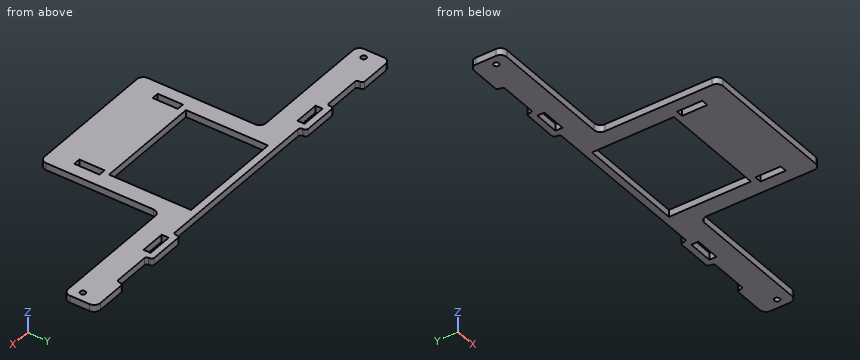
```python
from build123d import *

# Parameters (mm, degrees)
SKETCH_1_W               = 325
SKETCH_1_H               = 110
SKETCH_1_R               = 2.1
EXTRUDE_1_DEPTH          = 5.6
EXTRUDE_2_DEPTH          = 5.6
SKETCH_2_W               = 85
SKETCH_2_H               = 65
SKETCH_2_W_2             = 5.6
SKETCH_2_H_2             = 20
SKETCH_2_W_3             = 20
SKETCH_2_H_3             = 5.6
CUT_EXTRUDE_1_DEPTH      = 176.331029769
SKETCH_4_W               = 106.4
SKETCH_4_H               = 95
SKETCH_4_R               = 2.1
CUT_EXTRUDE_2_DEPTH      = 176.331029769
CUT_EXTRUDE_3_DEPTH      = 176.331029769
CUT_EXTRUDE_3_DEPTH_BACK = 176.331029769
SKETCH_5_W               = 140
SKETCH_5_H               = 5
SKETCH_5_W_2             = 32.5
FILLET_1_R               = 5
FILLET_2_R               = 2


with BuildPart() as part:
    # ｽｹｯﾁ1 → ﾎﾞｽ - 押し出し1 (new body)
    with BuildSketch(Plane.XY):
        Rectangle(SKETCH_1_W, SKETCH_1_H)
        with Locations((155, 50)):
            Circle(SKETCH_1_R, mode=Mode.SUBTRACT)
        with Locations(Location((155, -50, 0), (0, 0, 180))):
            Circle(SKETCH_1_R, mode=Mode.SUBTRACT)
        with Locations(Location((-155, 50, 0), (0, 0, 180))):
            Circle(SKETCH_1_R, mode=Mode.SUBTRACT)
        with Locations((-155, -50)):
            Circle(SKETCH_1_R, mode=Mode.SUBTRACT)
    extrude(amount=EXTRUDE_1_DEPTH)

    # ｽｹｯﾁ3 → ﾎﾞｽ - 押し出し2 (add)
    with BuildSketch(Plane.XY.offset(5.6)):
        Polygon((-162.5, 65.6), (-162.5, 55), (-95, 55), (-95, 60.6), (-75, 60.6), (-75, 55), (0, 55), (0, 65.6), align=None)
        Polygon((162.5, 65.6), (0, 65.6), (0, 55), (75, 55), (75, 60.6), (95, 60.6), (95, 55), (162.5, 55), align=None)
    extrude(amount=-EXTRUDE_2_DEPTH)

    # ｽｹｯﾁ2 → ｶｯﾄ - 押し出し1 (cut, through all)
    with BuildSketch(Plane.XY.offset(5.6)):
        with Locations((0, 22.5)):
            Rectangle(SKETCH_2_W, SKETCH_2_H)
        with Locations((-43.3, -25)):
            Rectangle(SKETCH_2_W_2, SKETCH_2_H_2)
        with Locations((43.3, -25)):
            Rectangle(SKETCH_2_W_2, SKETCH_2_H_2)
        with Locations((85, 57.8)):
            Rectangle(SKETCH_2_W_3, SKETCH_2_H_3)
        with Locations((-85, 57.8)):
            Rectangle(SKETCH_2_W_3, SKETCH_2_H_3)
    extrude(amount=-CUT_EXTRUDE_1_DEPTH, mode=Mode.SUBTRACT)

    # ｽｹｯﾁ4 → ｶｯﾄ - 押し出し2 (cut, through all)
    # profile 1 of 2: a face of its own
    with BuildSketch(Plane.XY.offset(5.6)):
        with Locations((-109.3, -7.5)):
            Rectangle(SKETCH_4_W, SKETCH_4_H)
        with Locations((-155, -50)):
            Circle(SKETCH_4_R, mode=Mode.SUBTRACT)
    # profile 2 of 2: a face of its own
    with BuildSketch(Plane.XY.offset(5.6)):
        with Locations((109.3, -7.5)):
            Rectangle(SKETCH_4_W, SKETCH_4_H)
        with Locations((155, -50)):
            Circle(SKETCH_4_R, mode=Mode.SUBTRACT)
    extrude(amount=-CUT_EXTRUDE_2_DEPTH, mode=Mode.SUBTRACT)

    # ｽｹｯﾁ5 → ｶｯﾄ - 押し出し3 (cut, two sides: drawn at the far end of the back side and taken through both)
    with BuildSketch(Plane.XY.offset(5.6).offset(-CUT_EXTRUDE_3_DEPTH_BACK)):
        with Locations((0, 63.1)):
            Rectangle(SKETCH_5_W, SKETCH_5_H)
        with Locations((-116.25, 63.1)):
            Rectangle(SKETCH_5_W_2, SKETCH_5_H)
        with Locations((116.25, 63.1)):
            Rectangle(SKETCH_5_W_2, SKETCH_5_H)
    extrude(amount=CUT_EXTRUDE_3_DEPTH + CUT_EXTRUDE_3_DEPTH_BACK, mode=Mode.SUBTRACT)

    # ﾌｨﾚｯﾄ1
    fillet_1_edges = [part.edges().sort_by_distance(p)[0] for p in [
        (-56.1, -55, 2.8),
        (-162.5, 40, 2.8),
        (-56.1, 40, 2.8),
        (162.5, 40, 2.8),
        (56.1, -55, 2.8),
        (56.1, 40, 2.8),
        (-162.5, 65.6, 2.8),
        (162.5, 65.6, 2.8),
    ]]
    fillet(fillet_1_edges, radius=FILLET_1_R)

    # ﾌｨﾚｯﾄ2
    fillet_2_edges = [part.edges().sort_by_distance(p)[0] for p in [
        (100, 65.6, 2.8),
        (132.5, 65.6, 2.8),
        (132.5, 60.6, 2.8),
        (100, 60.6, 2.8),
        (-132.5, 60.6, 2.8),
        (-132.5, 65.6, 2.8),
        (-100, 65.6, 2.8),
        (-100, 60.6, 2.8),
        (70, 65.6, 2.8),
        (70, 60.6, 2.8),
        (-70, 60.6, 2.8),
        (-70, 65.6, 2.8),
    ]]
    fillet(fillet_2_edges, radius=FILLET_2_R)


solid = part.part
```
Build history of the part. All positions in model axes, mm. Give positions to 0.01 mm unless a question says otherwise; leave off trailing zeros. Loops run counter-clockwise (first coordinate to the right, second up) from the corner with the lowest first, then second, coordinate; pieces in that order, holes last. Notation, with made-up numbers: (85, 57.25) -> (136, 57.25) arc R26 ccw to (136, 77.25) -> close; hole circle Ø3 at (48, -35.75). An arc over 180 degrees is marked (long way). One line per question, with ' | ' between items. Start each with the question number.
1) Cut at C-C (x = -141). Give the cut face in (y, z).
2) Cut at B-B (x = -12). Give the cut face in (y, z), plus the area to 3 significant figures.
3) Pin check, flat tips, straight feed: pin 1 (1.7 mm diameter, centred on x = -107.5, z = 3, fed in from -Y); pin 2 (1 mm diameter, centred on y = 40, z = 4, fed in from +X); pin 3 (3 mm diameter, centred on y = -28, z = 0.5, fed in from -X). Stop position of each tip, or through.
4) Cut at D-D (z = 4.6). Count the separate pieces of the cut face and the enclosed holes in it, plus the area to 3 significant figures.
5) Cut at A-A (y = 10). Give the cut face in (x, z).
6) Probe L1, parallel to X at y = 55.5, z = 3.8; L2, parallel to Y at x = -155, z = 3.2; L3, parallel to Y at x = -22, z = 2.9. List the from-to ranges inside material, lowest first.
Return value:
1) outline: (40, 0) -> (65.6, 0) -> (65.6, 5.6) -> (40, 5.6) -> close
2) outline: (-55, 0) -> (-10, 0) -> (-10, 5.6) -> (-55, 5.6) -> close; (55, 0) -> (60.6, 0) -> (60.6, 5.6) -> (55, 5.6) -> close | area: 283 mm^2
3) pin 1: y = 40 | pin 2: x = 159.68 | pin 3: x = -56.1
4) separate pieces: 1 | enclosed holes: 7 | area: 11,900 mm^2
5) outline: (-56.1, 0) -> (-42.5, 0) -> (-42.5, 5.6) -> (-56.1, 5.6) -> close; (42.5, 0) -> (56.1, 0) -> (56.1, 5.6) -> (42.5, 5.6) -> close
6) L1: -162.5 to -95, -75 to 75, 95 to 162.5 | L2: 40 to 47.9, 52.1 to 65.6 | L3: -55 to -10, 55 to 60.6
